The listing builds one solid part. Answer for the finished solid, in the listing's coordinates (mm). A direction names the side the tool comes from. Coordinates: 2 decimals unless noted, no trailing zeros. Write each loop counter-clockwise with the first axis right and the second up, starting at its lowest first coordinate (ties: lowest second). Pieces come first, ordered by that corner, then holes.
```python
from build123d import *

# Parameters (mm, degrees)
SKETCH1_R           = 14
BOSS_EXTRUDE1_DEPTH = 5


with BuildPart() as part:
    # Sketch1 → Boss-Extrude1 (new body)
    with BuildSketch(Plane(origin=(0, 0, 0), x_dir=(1, 0, 0), z_dir=(0, 1, 0))):
        with BuildLine():
            Line((-23.3, 4.4), (-10.5, 14))
            ThreePointArc((-10.5, 14), (0, 17.5), (10.5, 14))
            Line((10.5, 14), (23.3, 4.4))
            ThreePointArc((23.3, 4.4), (25.5, 0), (23.3, -4.4))
            Line((23.3, -4.4), (10.5, -14))
            ThreePointArc((10.5, -14), (0, -17.5), (-10.5, -14))
            Line((-10.5, -14), (-23.3, -4.4))
            ThreePointArc((-23.3, -4.4), (-25.5, 0), (-23.3, 4.4))
        make_face()
        with Locations(Location((0, 0, 0), (0, 0, 270))):
            Circle(SKETCH1_R, mode=Mode.SUBTRACT)
        Polygon((-20, 3.92598183), (-23.4, 1.962990915), (-23.4, -1.962990915), (-20, -3.92598183), (-16.6, -1.962990915), (-16.6, 1.962990915), align=None, mode=Mode.SUBTRACT)
        Polygon((20, -3.92598183), (23.4, -1.962990915), (23.4, 1.962990915), (20, 3.92598183), (16.6, 1.962990915), (16.6, -1.962990915), align=None, mode=Mode.SUBTRACT)
    extrude(amount=BOSS_EXTRUDE1_DEPTH)


solid = part.part
```
(1) Each of these flat-tipped pins is pushed along its axis until it touches: pin 1 (1 mm diameter, centred on x = -7.5, y = 4, fed in from -Z); pin 2 (3 mm diameter, centred on x = -19.5, y = 3.5, fed in from -Z) (3 decimals); pin 3 (1.2 mm diameter, centred on y = 3, z = -1, fed in from -X). Where does it stop, or does it pass through?
(2) For a pull along Z with two mould halves and no side action, classify faces 1 (the flat face through (21.724, 2.465, -2.931)), 2 (the flat face through (-16.81, 2.46, 9.27)), 3 (the flat face through (8, 5, -12)), 4 (the flat face through (21.676, 2.465, 2.958)) as pulls with the +Z half, pulls with the -Z half, needs draft (parallel to the pull), parting line crosses it, or undercut.
(3) Section B-B, the plane y = 0.5 is taken. Write down the section's boundary in (x, z).
(4) Which of the six approach directions +Z, -Z, +X, -X, +Y, -Y give full straight-line access (tool end or side, diameter ignored) to faces 5 (the flat face through (-21.724, 2.465, 2.931)), 6 (the flat face through (16.81, 2.46, -9.27))?
(5) Section D-D, the plane z = -11 is taken. Write down the section's boundary in (x, y), plus the area to 3 significant figures.
(6) Section C-C, the plane x = 0 is taken. Write down the section's boundary in (y, z).
(7) Section A-A, the plane z = 0 is taken. Write down the section's boundary in (x, y), plus the area to 3 significant figures.
(8) Find the intervals of material crossed by probe 1 along X at (y, z) = (4.35, 2); probe 2 along X at (y, z) = (2.45, 12.5); probe 3 along Z at (x, y) = (20, 0.85) (3 decimals), in increasing order.
Solution:
1. pin 1: stops at z = -16.04
1. pin 2: stops at z = -8.375
1. pin 3: stops at x = -25.49
2. face 1: undercut
2. face 2: pulls with the +Z half
2. face 3: needs draft
2. face 4: undercut
3. outline: (-23.3, -4.4) - (-10.5, -14) arc R17.5 ccw to (10.5, -14) - (23.3, -4.4) arc R5.5 ccw to (23.3, 4.4) - (10.5, 14) arc R17.5 ccw to (-10.5, 14) - (-23.3, 4.4) arc R5.5 ccw to start; hole (-23.4, -1.96) - (-20, -3.93) - (-16.6, -1.96) - (-16.6, 1.96) - (-20, 3.93) - (-23.4, 1.96) - close; hole circle Ø28 at (0, 0); hole (16.6, -1.96) - (20, -3.93) - (23.4, -1.96) - (23.4, 1.96) - (20, 3.93) - (16.6, 1.96) - close
4. face 5: +Y, -Y
4. face 6: -Z, +X, +Y, -Y
5. outline: (-14.5, 0) - (-8.66, 0) - (-8.66, 5) - (-14.5, 5) - close; (8.66, 0) - (14.5, 0) - (14.5, 5) - (8.66, 5) - close
5. area: 58.4 mm2
6. outline: (0, -17.5) - (5, -17.5) - (5, -14) - (0, -14) - close; (0, 14) - (5, 14) - (5, 17.5) - (0, 17.5) - close
7. outline: (-25.5, 0) - (-23.4, 0) - (-23.4, 5) - (-25.5, 5) - close; (-16.6, 0) - (-14, 0) - (-14, 5) - (-16.6, 5) - close; (14, 0) - (16.6, 0) - (16.6, 5) - (14, 5) - close; (23.4, 0) - (25.5, 0) - (25.5, 5) - (23.4, 5) - close
7. area: 47.0 mm2
8. probe 1: x = -25.12 to -23.34, -16.66 to -13.86, 13.86 to 16.66, 23.34 to 25.12
8. probe 2: x = -12.5 to -6.3, 6.3 to 12.5
8. probe 3: z = -6.875 to -3.926, 3.926 to 6.875
